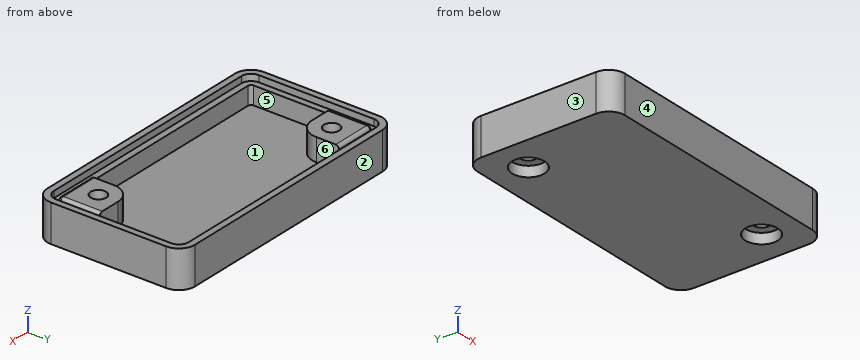
```python
from build123d import *

# Parameters (mm, degrees)
STOCK_PART3_1_START                              = -6
STOCK_PART3_1_DEPTH                              = 2
STOCK_PART3_1_START_2                            = -4
STOCK_PART3_1_2_DEPTH                            = 3.77
BOSS_EXTRUDE1_DEPTH                              = 3.5
CBORE_FOR_M2_PAN_HEAD_MACHINE_SCREW1_D           = 2.4
CBORE_FOR_M2_PAN_HEAD_MACHINE_SCREW1_CBORE_D     = 5
CBORE_FOR_M2_PAN_HEAD_MACHINE_SCREW1_CBORE_DEPTH = 1.6
CUT_EXTRUDE1_START                               = -1
CUT_EXTRUDE1_DEPTH                               = 1
FILLET1_R                                        = 0.5


# Read off the part's stored shape, not the designer's step: Stock-Part3-1
with BuildPart() as part:
    # Stock-Part3-1 outline → Stock-Part3-1 (new body)
    with BuildSketch(Plane.XY.offset(STOCK_PART3_1_START)):
        with BuildLine():
            Line((-36.200000763, -3), (0.5, -3))
            ThreePointArc((0.5, -3), (2.267766953, -2.267766953), (3, -0.5))
            Line((3, -0.5), (3, 17.299999237))
            ThreePointArc((3, 17.299999237), (2.267766953, 19.06776619), (0.5, 19.799999237))
            Line((0.5, 19.799999237), (-36.200000763, 19.799999237))
            ThreePointArc((-36.200000763, 19.799999237), (-37.967767716, 19.06776619), (-38.700000763, 17.299999237))
            Line((-38.700000763, 17.299999237), (-38.700000763, -0.5))
            ThreePointArc((-38.700000763, -0.5), (-37.967767716, -2.267766953), (-36.200000763, -3))
        make_face()
    extrude(amount=STOCK_PART3_1_DEPTH)

    # Stock-Part3-1 2 outline → Stock-Part3-1 2 (add)
    with BuildSketch(Plane.XY.offset(STOCK_PART3_1_START_2)):
        with BuildLine():
            Line((-36.200000763, -3), (0.5, -3))
            ThreePointArc((0.5, -3), (2.267766953, -2.267766953), (3, -0.5))
            Line((3, -0.5), (3, 17.299999237))
            ThreePointArc((3, 17.299999237), (2.267766953, 19.06776619), (0.5, 19.799999237))
            Line((0.5, 19.799999237), (-36.200000763, 19.799999237))
            ThreePointArc((-36.200000763, 19.799999237), (-37.967767716, 19.06776619), (-38.700000763, 17.299999237))
            Line((-38.700000763, 17.299999237), (-38.700000763, -0.5))
            ThreePointArc((-38.700000763, -0.5), (-37.967767716, -2.267766953), (-36.200000763, -3))
        make_face()
        with BuildLine():
            ThreePointArc((1, -0.5), (0.853553391, -0.853553391), (0.5, -1))
            Line((0.5, -1), (-36.200000763, -1))
            ThreePointArc((-36.200000763, -1), (-36.553554154, -0.853553391), (-36.700000763, -0.5))
            Line((-36.700000763, -0.5), (-36.700000763, 17.299999237))
            ThreePointArc((-36.700000763, 17.299999237), (-36.553554154, 17.653552628), (-36.200000763, 17.799999237))
            Line((-36.200000763, 17.799999237), (0.5, 17.799999237))
            ThreePointArc((0.5, 17.799999237), (0.853553391, 17.653552628), (1, 17.299999237))
            Line((1, 17.299999237), (1, -0.5))
        make_face(mode=Mode.SUBTRACT)
    extrude(amount=STOCK_PART3_1_2_DEPTH)

    # Sketch1 → Boss-Extrude1 (add)
    with BuildSketch(Plane.XY.offset(-4)):
        with BuildLine():
            Line((-33.200000683, 11.299999157), (-36.700000763, 11.299999157))
            Line((-36.700000763, 11.299999157), (-36.700000763, 17.299999237))
            ThreePointArc((-36.700000763, 17.299999237), (-36.553554154, 17.653552628), (-36.200000763, 17.799999237))
            Line((-36.200000763, 17.799999237), (-30.200000683, 17.799999237))
            Line((-30.200000683, 17.799999237), (-30.200000683, 14.299999157))
            ThreePointArc((-30.200000683, 14.299999157), (-31.078680339, 12.178678814), (-33.200000683, 11.299999157))
        make_face()
        with BuildLine():
            Line((-2.526751091, 5.473249069), (1, 5.473249069))
            Line((1, 5.473249069), (1, -0.5))
            ThreePointArc((1, -0.5), (0.853553391, -0.853553391), (0.5, -1))
            Line((0.5, -1), (-5.526751091, -1))
            Line((-5.526751091, -1), (-5.526751091, 2.473249069))
            ThreePointArc((-5.526751091, 2.473249069), (-4.648071434, 4.594569413), (-2.526751091, 5.473249069))
        make_face()
    extrude(amount=BOSS_EXTRUDE1_DEPTH)

    # CBORE for M2 Pan Head Machine Screw1 (through all)
    with Locations(Plane(origin=(0, 0, -6), x_dir=(-1, 0, 0), z_dir=(0, 0, -1))):
        with Locations((2.473250112, 2.526750908), (33.200000683, 14.299999157)):
            CounterBoreHole(CBORE_FOR_M2_PAN_HEAD_MACHINE_SCREW1_D / 2, CBORE_FOR_M2_PAN_HEAD_MACHINE_SCREW1_CBORE_D / 2, CBORE_FOR_M2_PAN_HEAD_MACHINE_SCREW1_CBORE_DEPTH)

    # Sketch4 → Cut-Extrude1 (cut)
    with BuildSketch(Plane.XY.offset(-0.23).offset(CUT_EXTRUDE1_START)):
        with BuildLine():
            Line((2, -0.5), (2, 17.299999237))
            ThreePointArc((2, 17.299999237), (1.560660172, 18.360659409), (0.5, 18.799999237))
            Line((0.5, 18.799999237), (-36.200000763, 18.799999237))
            ThreePointArc((-36.200000763, 18.799999237), (-37.260660935, 18.360659409), (-37.700000763, 17.299999237))
            Line((-37.700000763, 17.299999237), (-37.700000763, -0.5))
            ThreePointArc((-37.700000763, -0.5), (-37.260660935, -1.560660172), (-36.200000763, -2))
            Line((-36.200000763, -2), (0.5, -2))
            ThreePointArc((0.5, -2), (1.560660172, -1.560660172), (2, -0.5))
        make_face()
        with BuildLine():
            Line((1, -0.5), (1, 17.299999237))
            ThreePointArc((1, 17.299999237), (0.853553391, 17.653552628), (0.5, 17.799999237))
            Line((0.5, 17.799999237), (-36.200000763, 17.799999237))
            ThreePointArc((-36.200000763, 17.799999237), (-36.553554154, 17.653552628), (-36.700000763, 17.299999237))
            Line((-36.700000763, 17.299999237), (-36.700000763, -0.5))
            ThreePointArc((-36.700000763, -0.5), (-36.553554154, -0.853553391), (-36.200000763, -1))
            Line((-36.200000763, -1), (0.5, -1))
            ThreePointArc((0.5, -1), (0.853553391, -0.853553391), (1, -0.5))
        make_face(mode=Mode.SUBTRACT)
    extrude(amount=CUT_EXTRUDE1_DEPTH, mode=Mode.SUBTRACT)

    # Fillet1
    fillet1_edges = [part.edges().sort_by_distance(p)[0] for p in [
        (-33.200000723, 17.799999237, -0.5),
        (-36.553554154, 17.653552628, -0.5),
        (-36.700000763, 14.299999197, -0.5),
        (-2.513375545, -1, -0.5),
        (0.853553391, -0.853553391, -0.5),
        (1, 2.486624535, -0.5),
    ]]
    fillet(fillet1_edges, radius=FILLET1_R)


solid = part.part
```
The listing builds one solid part. Answer for the finished solid, in the listing's coordinates (mm). Face numbers are marked on the shaded views. A direction names the side the tool comes from. Give positions to 0.01 mm unless a question says otherwise; leave off trailing zeros. Order: outer loops, then holes, each group sorted by start corner. A loop starts at its lowest first (then second) coordinate and runs counter-clockwise, first axis right, second up. Notation, with made-up numbers: (80, 22.25) - (134, 22.25) arc R20 ccw to (134, 29.25) - close; hole circle Ø11 at (44, 28). An arc over 180 degrees is marked (long way). Use one line per item in the form item = value. Start each with the question number.
(1) A cutting plane is placed at C-C, the plane z = -4.85. Write down the section's boundary in (x, y).
(2) A cutting plane is placed at B-B, the plane y = 6. Write down the section's boundary in (x, z).
(3) For the marked faces 1 and 2, determine the directions among +Z, -Z, +X, -X, +Y, -Y from which every point of the face is accessible in a straight line to the end or side of a thin tool.
(4) Flat-ended cylindrical pins translate along their axes: pin 1 Ø6.5 at (x, y) = (-33.2, 14.3) entering from -Z; pin 2 Ø6.5 at (x, y) = (-33, 13.5) entering from +Z; pin 3 Ø3 at (x, y) = (-33.2, 14.3) entering from -Z. Find the tip coordinate at first contact, or state that the pin passes through.
(5) A cutting plane is placed at A-A, the plane x = -13.5. Write down the section's boundary in (y, z).
(6) A cutting plane is placed at D-D, the plane y = 3.25. Write down the section's boundary in (x, z).
(7) Consider line 1 (X direction, y = 14.3, z = -1.6); line 2 (Y direction, x = -11, z = -0.9); line 3 (Y direction, x = -9.5, z = -2.8). Determine where each line is inside the solid, lowest interval first. Write a range as from..to.
(8) The mould has two halves that part along X. Classify the marked faces 3, 4, 5 and 6: released by +X, released by -X, zero draft, split by the parting line, or undercut.
Ans:
q1.outline = (-38.7, -0.5) arc R2.5 ccw to (-36.2, -3) - (0.5, -3) arc R2.5 ccw to (3, -0.5) - (3, 17.3) arc R2.5 ccw to (0.5, 19.8) - (-36.2, 19.8) arc R2.5 ccw to (-38.7, 17.3) - close; hole circle Ø5 at (-33.2, 14.3); hole circle Ø5 at (-2.47, 2.53)
q2.outline = (-38.7, -6) - (3, -6) - (3, -0.23) - (2, -0.23) - (2, -1.23) - (1, -1.23) - (1, -4) - (-36.7, -4) - (-36.7, -1.23) - (-37.7, -1.23) - (-37.7, -0.23) - (-38.7, -0.23) - close
q3.face_1 = +Z
q3.face_2 = +Z, -Z, +X, -X, +Y
q4.pin_1 = -6
q4.pin_2 = -0.5
q4.pin_3 = -4.4
q5.outline = (-3, -6) - (19.8, -6) - (19.8, -0.23) - (18.8, -0.23) - (18.8, -1.23) - (17.8, -1.23) - (17.8, -4) - (-1, -4) - (-1, -1.23) - (-2, -1.23) - (-2, -0.23) - (-3, -0.23) - close
q6.outline = (-38.7, -6) - (-4.87, -6) - (-4.87, -4.4) - (-3.43, -4.4) - (-3.43, -0.5) - (-5.42, -0.5) - (-5.42, -4) - (-36.7, -4) - (-36.7, -1.23) - (-37.7, -1.23) - (-37.7, -0.23) - (-38.7, -0.23) - close; (-1.52, -4.4) - (-0.08, -4.4) - (-0.08, -6) - (3, -6) - (3, -0.23) - (2, -0.23) - (2, -1.23) - (1, -1.23) - (1, -1) arc R0.5 ccw to (0.5, -0.5) - (-1.52, -0.5) - close
q7.line_1 = -38.7..-34.4, -32..-30.2, 1..3
q7.line_2 = -3..-2, 18.8..19.8
q7.line_3 = -3..-1, 17.8..19.8
q8.face_3 = released by -X
q8.face_4 = zero draft
q8.face_5 = undercut
q8.face_6 = undercut
